from build123d import *

# Parameters (mm, degrees)
BOSS_EXTRUDE1_DEPTH = 50
SKETCH2_R           = 15
CUT_EXTRUDE1_DEPTH  = 50
CUT_EXTRUDE2_DEPTH  = 30


with BuildPart() as part:
    # Sketch1 → Boss-Extrude1 (new body)
    with BuildSketch(Plane.XY):
        with BuildLine():
            Line((-68.152842986, 0), (-68.152842986, 20))
            Line((-68.152842986, 20), (-42.152842986, 50))
            Line((-42.152842986, 50), (-38.152842986, 50))
            ThreePointArc((-38.152842986, 50), (-18.152842986, 30), (1.847157014, 50))
            Line((1.847157014, 50), (5.847157014, 50))
            Line((5.847157014, 50), (31.847157014, 20))
            Line((31.847157014, 20), (31.847157014, 0))
            Line((31.847157014, 0), (-68.152842986, 0))
        make_face()
    extrude(amount=-BOSS_EXTRUDE1_DEPTH)

    # Sketch2 → Cut-Extrude1 (cut)
    with BuildSketch(Plane(origin=(0, 50, 0), x_dir=(1, 0, 0), z_dir=(0, 1, 0))):
        with Locations(Location((-18.152842986, 25, 0), (0, 0, 180))):
            Circle(SKETCH2_R)
    extrude(amount=-CUT_EXTRUDE1_DEPTH, mode=Mode.SUBTRACT)

    # Sketch3 → Cut-Extrude2 (cut)
    with BuildSketch(Plane.XY.offset(-10)):
        Polygon((31.847157014, 0), (31.847157014, 20), (16.847157014, 37.307692308), (16.847157014, 0), align=None)
        Polygon((-68.152842986, 0), (-68.152842986, 20), (-53.152842986, 37.307692308), (-53.152842986, 0), align=None)
    extrude(amount=-CUT_EXTRUDE2_DEPTH, mode=Mode.SUBTRACT)


solid = part.part
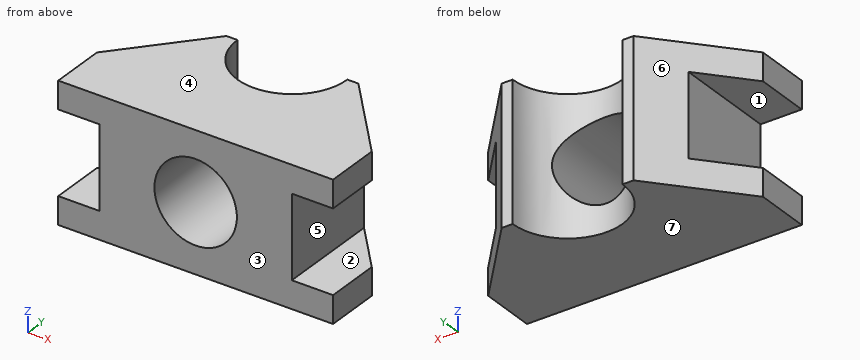
Input: part model. Units: mm. Frame: model coordinates. Face numbers are marked on the shaded views. A direction names the side the tool comes from. Round coordinates to 2 decimals unless told otherwise and drop trailing zeros. Loops run counter-clockwise (first coordinate to the right, second up) from the corner with the lowest first, then second, coordinate; pieces in that order, holes last. Notation, with made-up numbers: M 58.5,-24.75 L 109.5,-24.75 A13 cw 109.5,-18.75 Z; hole C 84.5,22 d7. An arc over 180 degrees is marked long. Answer as CSV lines item,"result". Start each with the question number.
(1) Section A-A, the plane z = -25. Output: boundary loops of the cut face in (x, y), plus the area to 3 significant figures.
(2) Section D-D, the plane z = -42. Output: boundary loops of the cut face in (x, y), plus the area to 3 significant figures.
(3) First-contact query: pin 1 (9 mm diameter, centred on y = 25, z = -28.5, fed in from +X); pin 2 (5 mm diameter, centred on y = 16.5, z = -30.5, fed in from -X). Flat tips, straight axial feed; report the tip coordinate or a pass-through.
(4) Reachability of the marked faces 1, 2 and 3 from +Z, -Z, +X, -X, +Y, -Y: full face, straight path, thin tool, end or side. Return the list, or none.
(5) Section C-C, the plane x = 20.5. Output: boundary loops of the cut face in (y, z).
(6) Section B-B, the plane y = 11. Output: boundary loops of the cut face in (x, z).
(7) Line query: line 1 (X direction, y = 13, z = -25); line 2 (Z direction, x = 20, y = 17.5); line 3 (Z direction, x = -12, y = 27). Output: solid intervals per line, ascending. Write a range as [from, to].
(8) Draft query along Z for the marked faces 4, 5, 6 and 7. Return one class per face: released by +Z, released by -Z, zero draft, split by the parting line, or undercut.
Values found:
1,outline,"M -53.15,0 L -33.15,0 L -33.15,36.77 A20 cw -38.15,50 L -42.15,50 L -53.15,37.31 Z; M -3.15,0 L 16.85,0 L 16.85,37.31 L 5.85,50 L 1.85,50 A20 cw -3.15,36.77 Z"
1,area,"1,770 mm²"
2,outline,"M -68.15,0 L 31.85,0 L 31.85,20 L 5.85,50 L 1.85,50 A20 cw -38.15,50 L -42.15,50 L -68.15,20 Z"
2,area,"3,590 mm²"
3,pin 1,"stops at x = 16.85"
3,pin 2,"stops at x = -53.15"
4,face 1,"-X, +Y, -Y"
4,face 2,"+X, +Y, -Y"
4,face 3,"+Z, -Z, +X, -X, -Y"
5,outline,"M 0,-50 L 33.09,-50 L 33.09,-40 L 0,-40 Z; M 0,-10 L 33.09,-10 L 33.09,0 L 0,0 Z"
6,outline,"M -68.15,-50 L 31.85,-50 L 31.85,-40 L 16.85,-40 L 16.85,-10 L 31.85,-10 L 31.85,0 L -68.15,0 L -68.15,-10 L -53.15,-10 L -53.15,-40 L -68.15,-40 Z; hole C -18.15,-25 d30"
7,line 1,"x = [-53.15, -33.15], [-3.15, 16.85]"
7,line 2,"z = [-50, -40], [-10, 0]"
7,line 3,"z = [-50, -38.68], [-11.32, 0]"
8,face 4,"released by +Z"
8,face 5,"undercut"
8,face 6,"zero draft"
8,face 7,"released by -Z"
